from build123d import *

# Parameters (mm, degrees)
F2_R = 5.08


with BuildPart() as f1:
    # F0 (on Front) → F1 (revolve)
    with BuildSketch(Plane.XZ):
        Polygon((0, 50.8), (0, 0), (4.932402, 12.7), (31.75, 9.240629), (31.75, 27.020629), (4.932402, 17.78), (4.932402, 50.8), align=None)
    revolve(axis=Axis((0, 0, 25.4), (0, 0, -1)))

    # F2
    f2_edges = [f1.edges().sort_by_distance(p)[0] for p in [
        (-31.75, 0, 9.240629),
        (-31.75, 0, 27.020629),
        (31.75, 0, 18.130629),
    ]]
    fillet(f2_edges, radius=F2_R)


solid = f1.part
Source: CAD feature listing. Evaluate the final solid. Frame: model axes, mm. A direction names the side the tool comes from. Give positions to 0.01 mm unless a question says otherwise; leave off trailing zeros. Write each loop counter-clockwise with the first axis right and the second up, starting at its lowest first coordinate (ties: lowest second). Pieces come first, ordered by that corner, then holes. Notation, with made-up numbers: M 79,74.25 L 89,74.25 A20 cw 89,81.25 Z; hole C 42.25,6.5 d11. An arc over 180 degrees is marked long. Return JSON: item names as keys, results as strings. Group by question number.
1) Pin query (flat end, axial travel): P1, Ø3, axis at y = 6.5, z = 26, coming from the +X side; P2, Ø1, axis at y = 16.5, z = 12.5, coming from the +X side; P3, Ø2, axis at x = 10.5, y = 19.5, coming from the -Z side. Return the tip coordinate at first contact, or that it passes through.
2) Cut plane B-B, the plane z = 22. Give the number of separate pieces and of enclosed holes in the cut face, plus the area to 3 significant figures.
3) Material intervals for line 1 along Z through (x, y) = (23, -14); line 2 along Z through (x, y) = (26.5, -12); line 3 along Y through (x, z) = (3.5, 37), sorted ascending. Write a range as [from, to].
4) Set-up query: faces 1 (the face through (4.7, -1.5, 34.5)), 2 (the face through (5.96, -1.88, 12.53)). Return all of +Z, -Z, +X, -X, +Y, -Y with unobstructed straight access to the full face (end or side cutting, diameter ignored); none if empty.
5) Cut plane A-A, the plane z = 40.5. Output: boundary loops of the cut face in (x, y).
6) Pull-direction query (X, two-part tool) for faces 3 (the face through (30.284, -9.537, 17.492)), 4 (the face through (0, 0, 50.8)), 5 (the face through (-0.4, 1.9, 5)); classes: pulls with the +X half, pulls with the -X half, needs draft (parallel to the pull), parting line crosses it, or undercut.
Recorded:
{
 "1": {"P1": "stops at x = 28.09", "P2": "stops at x = 26.77", "P3": "stops at z = 10.35"},
 "2": {"separate pieces": "2", "enclosed holes": "1", "area": "2,230 mm²"},
 "3": {"line 1": "z = [9.94, 24.97]", "line 2": "z = [10.55, 24.36]", "line 3": "y = [-3.48, 3.48]"},
 "4": {"face 1": "+Z", "face 2": "-Z"},
 "5": {"outline": "C 0,0 d9.86"},
 "6": {"face 3": "parting line crosses it", "face 4": "needs draft", "face 5": "undercut"}
}
